Source: CAD feature listing. Evaluate the final solid. Frame: model axes, mm. A direction names the side the tool comes from. Give positions to 0.01 mm unless a question says otherwise; leave off trailing zeros. Loops run counter-clockwise (first coordinate to the right, second up) from the corner with the lowest first, then second, coordinate; pieces in that order, holes last. Notation, with made-up numbers: (-21, 65) - (-3, 65) arc R15 ccw to (-3, 69) - close; hole circle Ø3 at (82.25, 88). An arc over 180 degrees is marked (long way). Put each result on its own line as item: value.
```python
from build123d import *

# Parameters (mm, degrees)
BOSS_EXTRUDE1_DEPTH = 10
SKETCH2_R           = 1.85
CUT_EXTRUDE1_DEPTH  = 20.697715604
SKETCH4_R           = 1.7
CUT_EXTRUDE2_DEPTH  = 20.697715604


with BuildPart() as part:
    # Sketch1 → Boss-Extrude1 (new body)
    with BuildSketch(Plane(origin=(0, 0, 0), x_dir=(0, 0, -1), z_dir=(1, 0, 0))):
        Polygon((-3, 12), (0, 12), (0, 0), (12, 0), (12, -3), (-3, -3), align=None)
    extrude(amount=BOSS_EXTRUDE1_DEPTH)

    # Sketch2 → Cut-Extrude1 (cut, through all)
    with BuildSketch(Plane(origin=(0, 0, 0), x_dir=(1, 0, 0), z_dir=(0, 1, 0))):
        with Locations(Location((5, 6, 0), (0, 0, 270))):
            Circle(SKETCH2_R)
    extrude(amount=-CUT_EXTRUDE1_DEPTH, mode=Mode.SUBTRACT)

    # Sketch4 → Cut-Extrude2 (cut, through all)
    with BuildSketch(Plane(origin=(0, 0, 0), x_dir=(-1, 0, 0), z_dir=(0, 0, -1))):
        with Locations((-5, 6)):
            Circle(SKETCH4_R)
    extrude(amount=-CUT_EXTRUDE2_DEPTH, mode=Mode.SUBTRACT)


solid = part.part
```
1) Pin query (flat end, axial travel): P1, Ø2, axis at x = 6.5, z = -4.5, coming from the +Y side; P2, Ø2, axis at x = 6, y = 6.5, coming from the -Z side. Return the tip coordinate at first contact, or that it passes through.
Check result:
P1: y = 0
P2: z = 0
2) Section query C-C, the plane x = 4. Output: boundary loops of the cut face in (y, z), plus the area to 3 significant figures.
Check result:
outline: (-3, -12) - (0, -12) - (0, -7.56) - (-3, -7.56) - close; (-3, -4.44) - (0, -4.44) - (0, 0) - (4.63, 0) - (4.63, 3) - (-3, 3) - close; (7.37, 0) - (12, 0) - (12, 3) - (7.37, 3) - close
area: 63.4 mm²
3) Access query for faces 4 (the cylindrical face through (5.37, 4.34, 1.48)), 5 (the flat face through (2.7, 0, -5.9)). Directions: +Z, -Z, +X, -X, +Y, -Y. A direction counts if a zero-diameter tool reaches every point of the face in a straight line with its end or side. Return the directions, or none.
Check result:
face 4: +Z, -Z
face 5: -Z, +X, -X, +Y
4) Section query B-B, the plane y = 6. Output: boundary loops of the cut face in (x, z), plus the area to 3 significant figures.
Check result:
outline: (0, 0) - (3.3, 0) - (3.3, 3) - (0, 3) - close; (6.7, 0) - (10, 0) - (10, 3) - (6.7, 3) - close
area: 19.8 mm²
5) Section query D-D, the plane z = 0.5. Output: boundary loops of the cut face in (x, y).
Check result:
outline: (0, -3) - (10, -3) - (10, 12) - (0, 12) - close; hole circle Ø3.4 at (5, 6)
6) Mould query, pull axis X, two halves, no side actions, for faces 1 (the flat face through (0, -0.4, -1.3)), 2 (the flat face through (5, 12, 2)), 3 (the cylindrical face through (5.08, -1.48, -7.85)). Classes: pulls with the +X half, pulls with the -X half, needs draft (parallel to the pull), parting line crosses it, or undercut.
Check result:
face 1: pulls with the -X half
face 2: needs draft
face 3: undercut
7) Material intervals for line 1 along X through (y, z) = (-0.8, -6); line 2 along Y through (x, z) = (5, 0.9); line 3 along Z through (x, y) = (8, 7), sorted ascending. Write a range as [from, to].
Check result:
line 1: [0, 3.15], [6.85, 10]
line 2: [-3, 4.3], [7.7, 12]
line 3: [0, 3]
8) Section query A-A, the plane z = -6. Output: boundary loops of the cut face in (x, y).
Check result:
outline: (0, -3) - (3.15, -3) - (3.15, 0) - (0, 0) - close; (6.85, -3) - (10, -3) - (10, 0) - (6.85, 0) - close
